The listing builds one solid part. Answer for the finished solid, in the listing's coordinates (mm). Face numbers are marked on the shaded views. A direction names the side the tool comes from. Round coordinates to 2 decimals unless told otherwise and drop trailing zeros. Order: outer loops, then holes, each group sorted by start corner. A loop starts at its lowest first (then second) coordinate and runs counter-clockwise, first axis right, second up. Notation, with made-up numbers: (56.25, 40.5) -> (94.25, 40.5) arc R15 cw to (94.25, 55.5) -> close; hole circle Ø3 at (45, 58). An arc over 180 degrees is marked (long way). Return JSON: item names as keys, results as strings. Group by question number.
(1) Determine the mould class of the marked faces 1, 2, 3 and 4 for opening direction X: +X half, -X half, draft (parallel to the pull), parting line (faces both ways), or undercut.
(2) Consider line 1 (Y direction, x = -7, z = 15.55); line 2 (Y direction, x = -8, z = 15.75); line 3 (Z direction, x = -19.5, y = 3). Determine where each line is inside the solid, lowest interval first. Write a range as [from, to].
(3) Each of these flat-tipped pins is pushed along its axis until it touches: pin 1 (6.5 mm diameter, centred on x = -12.38, y = 11.54, fed in from -Z); pin 2 (1 mm diameter, centred on y = 13, z = 15, fed in from -X); pin 3 (3.5 mm diameter, centred on y = 14.5, z = 15.5, fed in from +X); pin 4 (2 mm diameter, centred on x = 0.5, z = 11.5, fed in from -Y). Where does it stop, or does it pass through?
(4) The part is cut by section A-A (z = 14.5). Determine the outline of the cut face in (x, y), plus the area to 3 significant figures.
(5) Which of the six approach directions +Z, -Z, +X, -X, +Y, -Y give full straight-line access (tool end or side, diameter ignored) to the marked faces 5, 6, 7, 8 and 9?
(6) The part is cut by section D-D (y = 0). Determine the outline of the cut face in (x, z).
(7) The part is cut by section C-C (x = -7). Determine the outline of the cut face in (y, z), plus the area to 3 significant figures.
(8) The part is cut by section B-B (x = 4.5). Determine the outline of the cut face in (y, z).
from build123d import *

# Parameters (mm, degrees)
SKETCH1_R           = 8
SKETCH1_R_2         = 2
BOSS_EXTRUDE1_DEPTH = 3
SKETCH2_R           = 9.5
SKETCH2_R_2         = 8
BOSS_EXTRUDE2_DEPTH = 16.66
BOSS_EXTRUDE3_START = -3
SKETCH3_R           = 1.5
BOSS_EXTRUDE3_DEPTH = 3
FILLET1_R           = 3
FILLET2_R           = 1


with BuildPart() as part:
    # Sketch1 → Boss-Extrude1 (new body)
    with BuildSketch(Plane.XY):
        with BuildLine():
            Line((-20.074505522, -9.607669091), (-3.160038348, -15.764031671))
            ThreePointArc((-3.160038348, -15.764031671), (0.280834475, -15.613799919), (2.607669091, -13.074505522))
            Line((2.607669091, -13.074505522), (8.764031671, 3.839961652))
            ThreePointArc((8.764031671, 3.839961652), (8.613799919, 7.280834475), (6.074505522, 9.607669091))
            Line((6.074505522, 9.607669091), (-10.839961652, 15.764031671))
            ThreePointArc((-10.839961652, 15.764031671), (-14.280834475, 15.613799919), (-16.607669091, 13.074505522))
            Line((-16.607669091, 13.074505522), (-22.764031671, -3.839961652))
            ThreePointArc((-22.764031671, -3.839961652), (-22.613799919, -7.280834475), (-20.074505522, -9.607669091))
        make_face()
        with Locations((-7, 0)):
            Circle(SKETCH1_R, mode=Mode.SUBTRACT)
        with Locations((-12.379052297, 11.535414877)):
            Circle(SKETCH1_R_2, mode=Mode.SUBTRACT)
        with Locations((4.535414877, 5.379052297)):
            Circle(SKETCH1_R_2, mode=Mode.SUBTRACT)
        with Locations((-1.620947703, -11.535414877)):
            Circle(SKETCH1_R_2, mode=Mode.SUBTRACT)
        with Locations((-18.535414877, -5.379052297)):
            Circle(SKETCH1_R_2, mode=Mode.SUBTRACT)
    extrude(amount=BOSS_EXTRUDE1_DEPTH)

    # Sketch2 → Boss-Extrude2 (add)
    with BuildSketch(Plane.XY):
        with Locations(Location((-7, 0, 0), (0, 0, 180))):
            Circle(SKETCH2_R)
        with Locations((-7, 0)):
            Circle(SKETCH2_R_2, mode=Mode.SUBTRACT)
    extrude(amount=BOSS_EXTRUDE2_DEPTH)

    # Sketch3 → Boss-Extrude3 (add)
    # profile 1 of 2: a face of its own
    with BuildSketch(Plane.XY.offset(16.66).offset(BOSS_EXTRUDE3_START)):
        with BuildLine():
            Line((-4, 9.013878189), (-4, 17.5))
            ThreePointArc((-4, 17.5), (-7, 20.5), (-10, 17.5))
            Line((-10, 17.5), (-10, 9.013878189))
            ThreePointArc((-10, 9.013878189), (-7, 9.5), (-4, 9.013878189))
        make_face()
        with Locations((-7, 17.5)):
            Circle(SKETCH3_R, mode=Mode.SUBTRACT)
    # profile 2 of 2: a face of its own
    with BuildSketch(Plane.XY.offset(16.66).offset(BOSS_EXTRUDE3_START)):
        with BuildLine():
            Line((-10, -9.013878189), (-10, -17.5))
            ThreePointArc((-10, -17.5), (-7, -20.5), (-4, -17.5))
            Line((-4, -17.5), (-4, -9.013878189))
            ThreePointArc((-4, -9.013878189), (-7, -9.5), (-10, -9.013878189))
        make_face()
        with Locations((-7, -17.5)):
            Circle(SKETCH3_R, mode=Mode.SUBTRACT)
    extrude(amount=BOSS_EXTRUDE3_DEPTH)

    # Fillet1
    fillet1_edges = [part.edges().sort_by_distance(p)[0] for p in [
        (-10, -9.013878189, 15.16),
        (-4, -9.013878189, 15.16),
        (-7, -9.5, 13.66),
        (-4, 9.013878189, 15.16),
        (-10, 9.013878189, 15.16),
        (-7, 9.5, 13.66),
    ]]
    fillet(fillet1_edges, radius=FILLET1_R)

    # Fillet2
    fillet2_edges = [part.edges().sort_by_distance(p)[0] for p in [
        (2.5, 0, 3),
    ]]
    fillet(fillet2_edges, radius=FILLET2_R)


solid = part.part
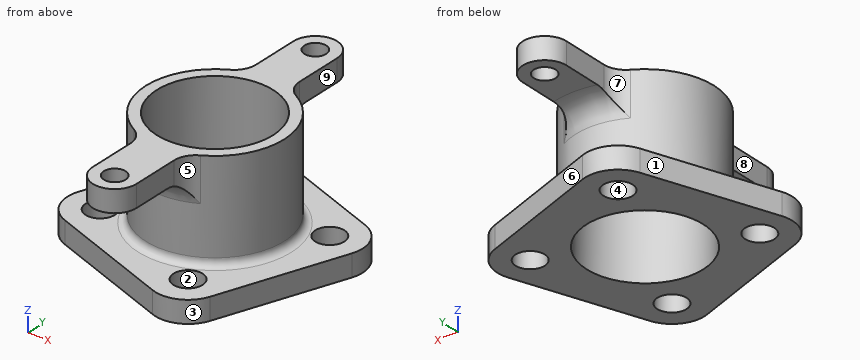
Answer below:
{
 "1": {"face 1": "-X half", "face 2": "undercut", "face 3": "parting line", "face 4": "undercut"},
 "2": {"line 1": "y = [-20.5, -19], [-16, -8], [8, 16], [19, 20.5]", "line 2": "y = [-20.33, -18.62], [-16.38, -7.94], [7.94, 16.38], [18.62, 20.33]", "line 3": "z = [0, 3]"},
 "3": {"pin 1": "stops at z = 0", "pin 2": "stops at x = -10", "pin 3": "stops at x = -4", "pin 4": "stops at y = -6.93"},
 "4": {"outline": "(-11.56, -8.33) arc R3 cw to (-10, -10.97) -> (-10, -17.5) arc R3 ccw to (-4, -17.5) -> (-4, -10.97) arc R3 cw to (-2.44, -8.33) arc R9.5 ccw to (-2.44, 8.33) arc R3 cw to (-4, 10.97) -> (-4, 17.5) arc R3 ccw to (-10, 17.5) -> (-10, 10.97) arc R3 cw to (-11.56, 8.33) arc R9.5 ccw to start; hole circle Ø16 at (-7, 0); hole circle Ø3 at (-7, -17.5); hole circle Ø3 at (-7, 17.5)", "area": "197 mm²"},
 "5": {"face 5": "+Z, +X, -Y", "face 6": "-Z, +X, +Y", "face 7": "+Z, -X, +Y", "face 8": "+Z, -X, -Y", "face 9": "+Z, +X, +Y"},
 "6": {"outline": "(-21.37, 0) -> (-15, 0) -> (-15, 16.66) -> (-16.5, 16.66) -> (-16.5, 4) arc R1 cw to (-17.5, 3) -> (-21.37, 3) -> close; (1, 0) -> (7.37, 0) -> (7.37, 3) -> (3.5, 3) arc R1 cw to (2.5, 4) -> (2.5, 16.66) -> (1, 16.66) -> close"},
 "7": {"outline": "(-20.5, 13.66) -> (-19, 13.66) -> (-19, 16.66) -> (-20.5, 16.66) -> close; (-16, 13.66) -> (-12.5, 13.66) arc R3 cw to (-9.5, 10.66) -> (-9.5, 4) arc R1 cw to (-10.5, 3) -> (-14.37, 3) -> (-14.37, 0) -> (-8, 0) -> (-8, 16.66) -> (-16, 16.66) -> close; (8, 0) -> (14.37, 0) -> (14.37, 3) -> (10.5, 3) arc R1 cw to (9.5, 4) -> (9.5, 10.66) arc R3 cw to (12.5, 13.66) -> (16, 13.66) -> (16, 16.66) -> (8, 16.66) -> close; (19, 13.66) -> (20.5, 13.66) -> (20.5, 16.66) -> (19, 16.66) -> close", "area": "131 mm²"},
 "8": {"outline": "(-7.88, 0) -> (3.38, 0) -> (3.38, 3) -> (-7.88, 3) -> close; (7.38, 0) -> (10.18, 0) -> (10.18, 3) -> (7.38, 3) -> close"}
}
